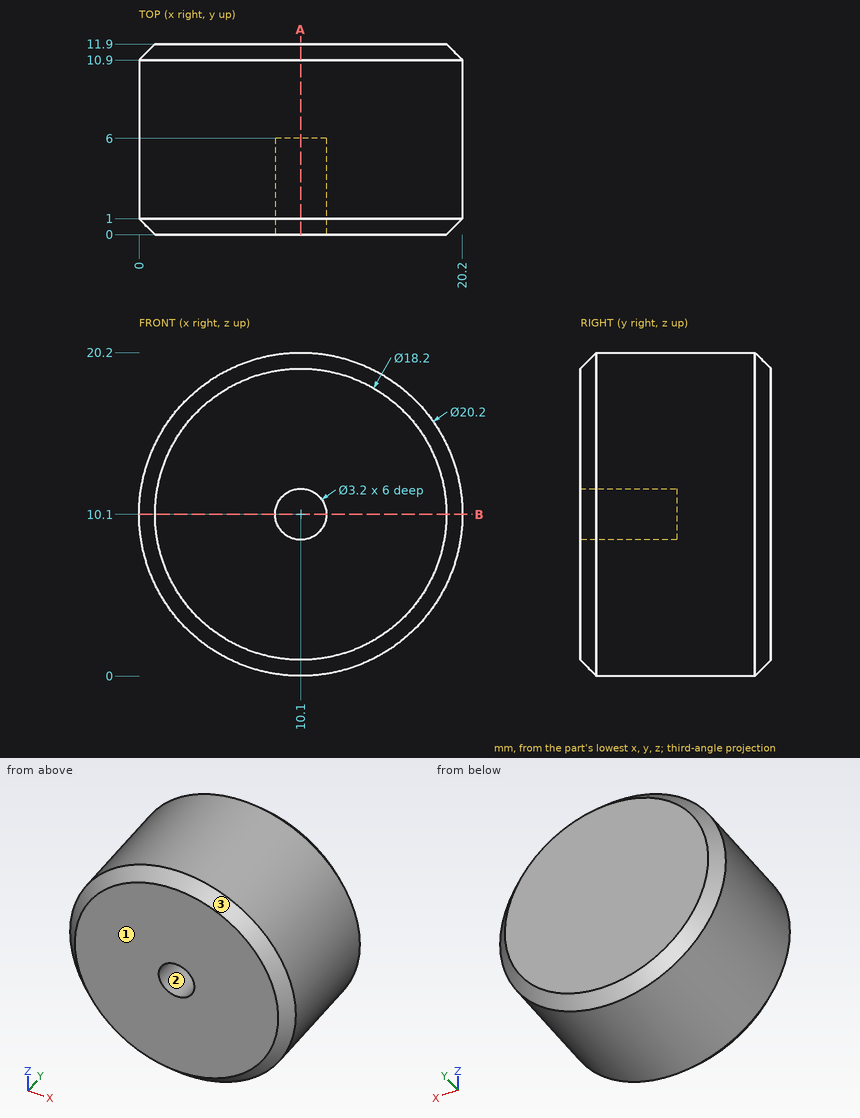
Part print with two shaded views. Sizes in mm from the minimum x, y, z corner. Round coordinates to 2 decimals unless told otherwise and drop trailing zeros. Order: outer loops, then holes, each group sorted by start corner. A loop starts at its lowest first (then second) coordinate and runs counter-clockwise, first axis right, second up. Notation, with made-up numbers: M 67.25,-34.5 L 120.25,-34.5 A36 ccw 120.25,4.5 Z; hole C 40.5,81.25 d8. An arc over 180 degrees is marked long. Answer in a Markdown table with one row per item. Add a question column.
Q1. Mould opens along X. For the marked faces 1, 2 and 3 say: +X half, -X half, draft (parallel to the pull), parting line (faces both ways), or undercut.
Q2. Pin check, flat tips, straight feed: pin 1 (3 mm diameter, centred on y = 3.5, z = 2.5, fed in from +X); pin 2 (5 mm diameter, centred on y = 1.5, z = 16.5, fed in from +X); pin 3 (1.9 mm diameter, centred on x = 10.1, z = 10.1, fed in from -Y). Stop position of each tip, or through.
Q3. Cut at A-A on x = 10.1. Give the cut face in (y, z), and give its area (3 significant figures).
Q4. Wall check: L1, parallel to X at y = 3.9, z = 10.1; L2, parallel to Y at x = 8.75, z = 10.75. Give the ranges that are in metal, low to high. Write a range as from..to.
Q5. Cut at B-B on z = 10.1. Give the cut face in (x, y).
Established:
| question | item | result |
|---|---|---|
| 1 | face 1 | draft |
| 1 | face 2 | undercut |
| 1 | face 3 | parting line |
| 2 | pin 1 | stops at x = 18.15 |
| 2 | pin 2 | stops at x = 19.42 |
| 2 | pin 3 | stops at y = 6 |
| 3 | outline | M 0,1 L 1,0 L 10.9,0 L 11.9,1 L 11.9,19.2 L 10.9,20.2 L 1,20.2 L 0,19.2 L 0,11.7 L 6,11.7 L 6,8.5 L 0,8.5 Z |
| 3 | area | 219 mm2 |
| 4 | L1 | x = 0..8.5, 11.7..20.2 |
| 4 | L2 | y = 6..11.9 |
| 5 | outline | M 0,1 L 1,0 L 8.5,0 L 8.5,6 L 11.7,6 L 11.7,0 L 19.2,0 L 20.2,1 L 20.2,10.9 L 19.2,11.9 L 1,11.9 L 0,10.9 Z |
